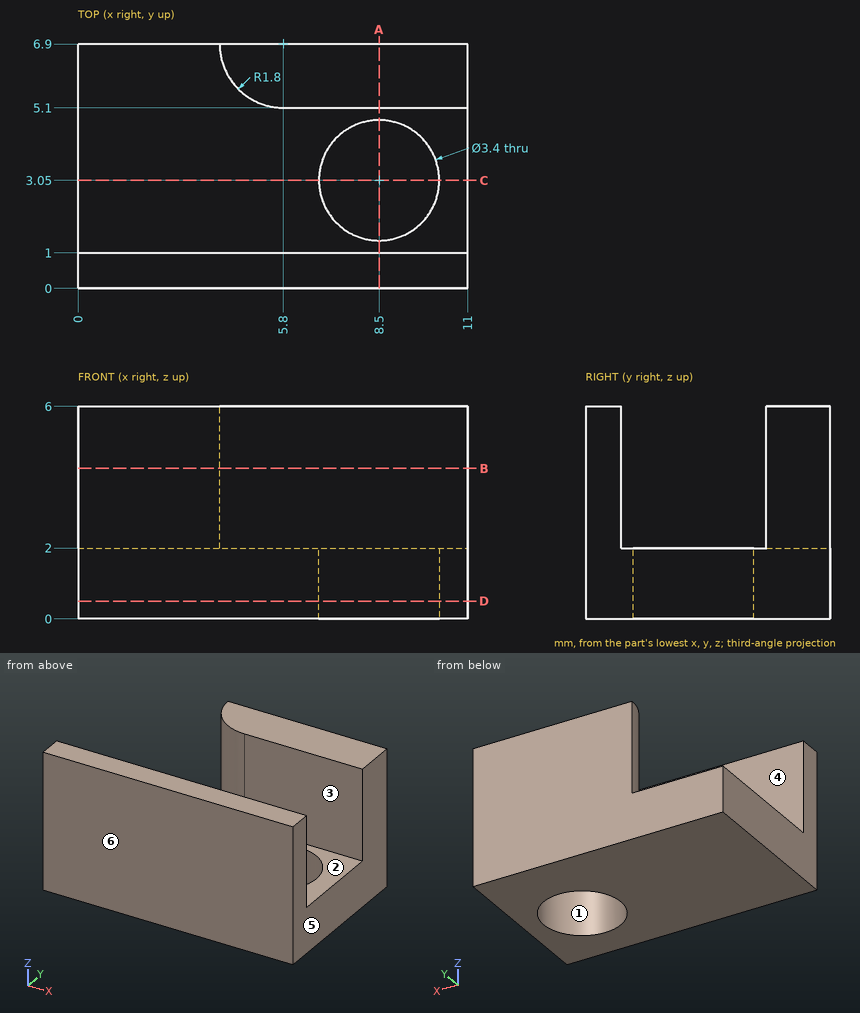
The figure shows three views and two pictorial views of one solid part (mm, origin at its lowest corner). Answer the questions. A direction names the side the tool comes from. Give positions to 0.01 mm unless a question says otherwise; leave off trailing zeros. Loops run counter-clockwise (first coordinate to the right, second up) from the corner with the lowest first, then second, coordinate; pieces in that order, holes last. Notation, with made-up numbers: (-23, 12.25) - (-4, 12.25) arc R19 ccw to (-4, 36.25) - close; hole circle Ø7 at (23, -21). An arc over 180 degrees is marked (long way). Answer in a Markdown table with one row per item.
(1) A tool of negligible diameter and unlimited length cuts with its end or side. For the marked faces 1, 2 and 3, from which of +Z, -Z, +X, -X, +Y, -Y can it reach the whole face along a straight path? Write none if from no direction.
Results list:
| item | result |
|---|---|
| face 1 | +Z, -Z |
| face 2 | +Z, -X |
| face 3 | +Z, +X, -X |
(2) Section C-C (y = 3.05) is taken. Give the vertices of the cut face in (x, z).
Results list:
| item | result |
|---|---|
| outline | (0, 0) - (6.8, 0) - (6.8, 2) - (0, 2) - close; (10.2, 0) - (11, 0) - (11, 2) - (10.2, 2) - close |
(3) For a pull along Y with two mould halves and no side action, classify the marked faces 4, 5 and 6 as pulls with the +Y half, pulls with the -Y half, needs draft (parallel to the pull), parting line crosses it, or undercut.
Results list:
| item | result |
|---|---|
| face 4 | undercut |
| face 5 | needs draft |
| face 6 | pulls with the -Y half |
(4) Section A-A (x = 8.5) is taken. Give the vertices of the cut face in (y, z), and give its area (3 significant figures).
Results list:
| item | result |
|---|---|
| outline | (0, 0) - (1.35, 0) - (1.35, 2) - (1, 2) - (1, 6) - (0, 6) - close; (4.75, 0) - (6.9, 0) - (6.9, 6) - (5.1, 6) - (5.1, 2) - (4.75, 2) - close |
| area | 18.2 mm² |
(5) Consider L1, parallel to X at y = 3, z = 1.5; L2, parallel to Y at x = 6.75, z = 3.5; L3, parallel to Y at x = 1, z = 5.15. Determine where each line is inside the solid, lowest interval first. Write a range as [from, to].
Results list:
| item | result |
|---|---|
| L1 | x = [0, 6.8], [10.2, 11] |
| L2 | y = [0, 1], [5.1, 6.9] |
| L3 | y = [0, 1] |
(6) Section D-D (z = 0.5) is taken. Give the vertices of the cut face in (x, y).
Results list:
| item | result |
|---|---|
| outline | (0, 0) - (11, 0) - (11, 6.9) - (0, 6.9) - close; hole circle Ø3.4 at (8.5, 3.05) |
(7) A flat-ended cylindrical pin translates along its axis: pin 1 Ø2 at (x, y) = (8.5, 3.05) entering from -Z. Find the tip coordinate at first contact, or state that the pin passes through.
Results list:
| item | result |
|---|---|
| pin 1 | passes through |
(8) Section B-B (z = 4.25) is taken. Give the vertices of the cut face in (x, y), and give its area (3 significant figures).
Results list:
| item | result |
|---|---|
| outline | (0, 0) - (11, 0) - (11, 1) - (0, 1) - close; (4, 6.9) arc R1.8 ccw to (5.8, 5.1) - (11, 5.1) - (11, 6.9) - close |
| area | 22.9 mm² |
